Model file for the job. Use its own axes, mm. Give positions to 0.01 mm unless a question says otherwise; leave off trailing zeros. Write each loop counter-clockwise with the first axis right and the second up, starting at its lowest first coordinate (ties: lowest second). Pieces come first, ordered by that corner, then holes. Notation, with made-up numbers: (3, -36) - (46, -36) arc R32 ccw to (46, 2) - close; hole circle Ø8 at (32, -28.5). An arc over 180 degrees is marked (long way). One line per item, written item: value. Start each with the question number.
(1) Probe L1, parallel to X at y = -2.2, z = 7.5; L2, parallel to Z at x = 15, y = -3.3; L3, parallel to Z at x = 17, y = -3. List the from-to ranges inside material, lowest first.
(2) Cut at A-A, the plane y = -1.2. List the corners of the cut face in (x, z) (3 decimals), and give its area (3 significant figures).
(3) Cut at B-B, the plane z = 9.5. List the corners of the cut face in (x, y).
(4) Drop flat-ended pins along their axis: P1, Ø1.2, axis at x = 11, y = -3, coming from the +Z side; P2, Ø1, axis at y = -2, z = 15.5, coming from the -X side. Give the stop position or say it passes through.
(5) Cut at C-C, the plane z = -3. List the corners of the cut face in (x, y).
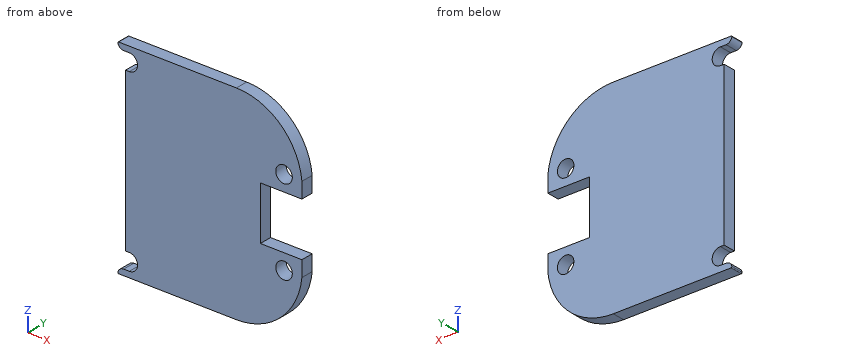
from build123d import *

# Parameters (mm, degrees)
F0_W     = 68.523422
F0_H     = 74.860842
F1_DEPTH = 4
F2_R     = 2.63906
F3_DEPTH = 4.001
F4_W     = 1.2
F4_H     = 50.72188
F5_DEPTH = 4
F6_R     = 0.254


with BuildPart() as f1:
    # F0 (on Front) → F1 (new body)
    with BuildSketch(Plane.XZ):
        Rectangle(F0_W, F0_H)
    extrude(amount=F1_DEPTH)

    # F2 (on face) → F3 (cut, through all)
    with BuildSketch(Plane.XZ.offset(4)):
        with Locations((-34.261711, 28)):
            Circle(F2_R)
        with Locations((15.238289, 13.5)):
            Circle(F2_R)
        with Locations((-34.261711, -28)):
            Circle(F2_R)
        with Locations((15.238289, -13.5)):
            Circle(F2_R)
        with BuildLine():
            Line((20.95, 8.5), (7.638289, 8.5))
            Line((7.638289, 8.5), (7.638289, 0))
            Line((7.638289, 0), (34.261711, 0))
            Line((34.261711, 0), (34.261711, 8.5))
            Line((34.261711, 8.5), (34.261711, 37.430421))
            Line((34.261711, 37.430421), (-34.261711, 37.430421))
            Line((-34.261711, 37.430421), (-34.261711, 32.5))
            Line((-34.261711, 32.5), (0, 32.5))
            ThreePointArc((0, 32.5), (14.141274, 27.042549), (20.95, 13.5))
            Line((20.95, 13.5), (20.95, 8.5))
        make_face()
        with BuildLine():
            Line((34.261711, 0), (7.638289, 0))
            Line((7.638289, 0), (7.638289, -8.5))
            Line((7.638289, -8.5), (20.95, -8.5))
            Line((20.95, -8.5), (20.95, -13.5))
            ThreePointArc((20.95, -13.5), (14.141274, -27.042549), (0, -32.5))
            Line((0, -32.5), (-34.261711, -32.5))
            Line((-34.261711, -32.5), (-34.261711, -37.430421))
            Line((-34.261711, -37.430421), (34.261711, -37.430421))
            Line((34.261711, -37.430421), (34.261711, -8.5))
            Line((34.261711, -8.5), (34.261711, 0))
        make_face()
    extrude(amount=-F3_DEPTH, mode=Mode.SUBTRACT)

    # F4 (on face) → F5 (join, through all)
    with BuildSketch(Plane.XZ.offset(4)):
        with BuildLine():
            Line((-34.261711, -32.5), (-34.261711, -30.63906))
            Line((-34.261711, -30.63906), (-36.061711, -30.63906))
            ThreePointArc((-36.061711, -30.63906), (-37.393081, -31.181533), (-37.966201, -32.5))
            Line((-37.966201, -32.5), (-34.261711, -32.5))
        make_face()
        with Locations((-34.861711, 0)):
            Rectangle(F4_W, F4_H)
        with BuildLine():
            Line((-36.061711, 30.63906), (-34.261711, 30.63906))
            Line((-34.261711, 30.63906), (-34.261711, 32.5))
            Line((-34.261711, 32.5), (-37.966201, 32.5))
            ThreePointArc((-37.966201, 32.5), (-37.393081, 31.181533), (-36.061711, 30.63906))
        make_face()
    extrude(amount=-F5_DEPTH)

    # F6
    f6_edges = [f1.edges().sort_by_distance(p)[0] for p in [
        (-37.966201, -2, -32.5),
        (-37.966201, -2, 32.5),
    ]]
    fillet(f6_edges, radius=F6_R)


solid = f1.part
Answers follow:
1. L1: x = -35.46 to 7.64
1. L2: z = -26.22 to -16.13, -10.87 to -8.5, 8.5 to 10.87, 16.13 to 26.22
1. L3: z = -23.86 to -15.46, -11.54 to -8.5, 8.5 to 11.54, 15.46 to 23.86
2. outline: (-37.935, -32.2) arc R0.254 ccw to (-37.686, -32.5) - (0, -32.5) arc R21.05 ccw to (20.95, -13.5) - (20.95, -8.5) - (7.638, -8.5) - (7.638, 8.5) - (20.95, 8.5) - (20.95, 13.5) arc R21.05 ccw to (0, 32.5) - (-37.686, 32.5) arc R0.254 ccw to (-37.935, 32.2) arc R1.905 ccw to (-36.062, 30.639) - (-34.262, 30.639) arc R2.639 cw to (-34.262, 25.361) - (-35.462, 25.361) - (-35.462, -25.361) - (-34.262, -25.361) arc R2.639 cw to (-34.262, -30.639) - (-36.062, -30.639) arc R1.905 ccw to start; hole circle Ø5.278 at (15.238, -13.5); hole circle Ø5.278 at (15.238, 13.5)
2. area: 3,180 mm²
3. outline: (-35.46, -4) - (20.95, -4) - (20.95, 0) - (-35.46, 0) - close
4. P1: stops at z = 29.75
4. P2: stops at x = -35.46
5. outline: (-35.46, -4) - (7.64, -4) - (7.64, 0) - (-35.46, 0) - close
